```python
from build123d import *

# Parameters (mm, degrees)
SKETCH1_W                      = 200
SKETCH1_H                      = 300
BOSS_EXTRUDE1_DEPTH            = 4.7625
CUT_EXTRUDE1_DEPTH             = 181.340459704
SKETCH15_R                     = 3.5
BOSS_EXTRUDE2_DEPTH            = 4.7625
M3X0_5_TAPPED_HOLE3_D          = 2.5
M5_CLEARANCE_HOLE1_D           = 5.3
FILLET2_R                      = 3
M3X0_5_TAPPED_HOLE4_AT_2_COUNT = 2
M3X0_5_TAPPED_HOLE4_AT_2_PITCH = 150
M3X0_5_TAPPED_HOLE5_AT_2_COUNT = 2
M3X0_5_TAPPED_HOLE5_AT_2_PITCH = 137.5
M3X0_5_TAPPED_HOLE5_AT_3_COUNT = 2
M3X0_5_TAPPED_HOLE5_AT_3_PITCH = 275
FILLET1_R                      = 1


with BuildPart() as part:
    # Sketch1 → Boss-Extrude1 (new body)
    with BuildSketch(Plane(origin=(0, 0, 0), x_dir=(1, 0, 0), z_dir=(0, 1, 0))):
        Rectangle(SKETCH1_W, SKETCH1_H)
    extrude(amount=BOSS_EXTRUDE1_DEPTH)

    # Sketch14 → Cut-Extrude1 (cut, through all)
    with BuildSketch(Plane(origin=(0, 4.7625, 0), x_dir=(1, 0, 0), z_dir=(0, 1, 0))):
        Polygon((-83.751800259, 15), (83.751800259, 15), (0, -54.793166883), align=None)
        Polygon((90, 9.793166883), (90, -129.793166883), (6.248199741, -60), align=None)
        Polygon((83.751800259, -135), (-83.751800259, -135), (0, -65.206833117), align=None)
        Polygon((-90, -129.793166883), (-90, 9.793166883), (-6.248199741, -60), align=None)
        with BuildLine():
            Line((8.236504113, 90), (90, 135.424164382))
            Line((90, 135.424164382), (90, 128))
            ThreePointArc((90, 128), (87, 125), (90, 122))
            Line((90, 122), (90, 70))
            ThreePointArc((90, 70), (87, 67), (90, 64))
            Line((90, 64), (90, 44.575835618))
            Line((90, 44.575835618), (59.796175629, 61.355738047))
            Line((59.796175629, 61.355738047), (62.122471828, 65.543071206))
            ThreePointArc((62.122471828, 65.543071206), (60.956928794, 69.622471828), (56.877528172, 68.456928794))
            Line((56.877528172, 68.456928794), (54.551231972, 64.269595634))
            Line((54.551231972, 64.269595634), (8.236504113, 90))
        make_face()
        Polygon((81.763495887, 140), (0, 94.575835618), (-81.763495887, 140), align=None)
        Polygon((-90, 135.424164382), (-8.236504113, 90), (-90, 44.575835618), align=None)
        Polygon((-81.763495887, 40), (0, 85.424164382), (81.763495887, 40), align=None)
    extrude(amount=-CUT_EXTRUDE1_DEPTH, mode=Mode.SUBTRACT)

    # Sketch15 → Boss-Extrude2 (add)
    with BuildSketch(Plane(origin=(0, 4.7625, 0), x_dir=(1, 0, 0), z_dir=(0, 1, 0))):
        with Locations((85, -140)):
            Circle(SKETCH15_R)
    extrude(amount=-BOSS_EXTRUDE2_DEPTH)

    # M3x0.5 Tapped Hole3 (through all)
    with Locations(Plane(origin=(0, 4.7625, 0), x_dir=(1, 0, 0), z_dir=(0, 1, 0))):
        with Locations((85, 17.25), (-47, 17.25), (85, -140), (-70, -140), (-92, 145), (-92, 35), (43, 35), (43, 145), (59.5, 67), (90, 67), (90, 125), (59.5, 125)):
            Hole(M3X0_5_TAPPED_HOLE3_D / 2)

    # M5 Clearance Hole1 (through all)
    with Locations(Plane(origin=(0, 4.7625, 0), x_dir=(1, 0, 0), z_dir=(0, 1, 0))):
        with Locations((-95, 62.5), (-95, -62.5), (95, -62.5), (95, 62.5)):
            Hole(M5_CLEARANCE_HOLE1_D / 2)

    # Sketch29 → CSK for M5 Flat Head Machine Screw1 (revolve, cut)
    with BuildSketch(Plane(origin=(95, 4.7625, 62.5), x_dir=(0, 0, 1), z_dir=(1, 0, 0))):
        Polygon((0, 0), (0, 4.7625), (2.65, 4.7625), (2.65, 2.55), (5.2, 0), align=None)
    revolve(axis=Axis((95, 11.1125, 62.5), (0, -1, 0)), mode=Mode.SUBTRACT)

    # Fillet2
    fillet2_edges = [part.edges().sort_by_distance(p)[0] for p in [
        (6.248199741, 2.38125, 60),
        (90, 2.38125, -9.793166883),
        (90, 2.38125, 129.793166883),
        (54.551231972, 2.38125, -64.269595634),
        (8.236504113, 2.38125, -90),
        (90, 2.38125, -135.424164382),
        (90, 2.38125, -128),
        (90, 2.38125, -122),
        (90, 2.38125, -70),
        (90, 2.38125, -64),
        (90, 2.38125, -44.575835618),
        (59.796175629, 2.38125, -61.355738047),
        (-6.248199741, 2.38125, 60),
        (-90, 2.38125, 129.793166883),
        (-90, 2.38125, -9.793166883),
        (0, 2.38125, 54.793166883),
        (-83.751800259, 2.38125, -15),
        (83.751800259, 2.38125, -15),
        (0, 2.38125, 65.206833117),
        (83.751800259, 2.38125, 135),
        (-83.751800259, 2.38125, 135),
        (81.763495887, 2.38125, -40),
        (-81.763495887, 2.38125, -40),
        (0, 2.38125, -85.424164382),
        (-90, 2.38125, -44.575835618),
        (-90, 2.38125, -135.424164382),
        (-8.236504113, 2.38125, -90),
        (-81.763495887, 2.38125, -140),
        (81.763495887, 2.38125, -140),
        (0, 2.38125, -94.575835618),
    ]]
    fillet(fillet2_edges, radius=FILLET2_R)

    # Sketch22 → M3x0.5 Tapped Hole4 (revolve, cut)
    with BuildSketch(Plane(origin=(-75, 2.38125, 150), x_dir=(0, -1, 0), z_dir=(1, 0, 0))):
        Polygon((0, 0), (0, 10.751075774), (1.25, 10), (1.25, 0), align=None)
    m3x0_5_tapped_hole4 = revolve(axis=Axis((-75, 2.38125, 156.35), (0, 0, -1)), mode=Mode.SUBTRACT)

    # M3x0.5 Tapped Hole4 at 2: M3x0.5 Tapped Hole4 ×2
    with Locations(*[(i * M3X0_5_TAPPED_HOLE4_AT_2_PITCH, 0, 0) for i in range(1, M3X0_5_TAPPED_HOLE4_AT_2_COUNT)]):
        add(m3x0_5_tapped_hole4, mode=Mode.SUBTRACT)

    # Mirror1: M3x0.5 Tapped Hole4 across plane
    add(m3x0_5_tapped_hole4.mirror(Plane.XY), mode=Mode.SUBTRACT)

    # Mirror1 copy 1 sketch → Mirror1 copy 1 (revolve, cut)
    with BuildSketch(Plane(origin=(75, 2.38125, -150), x_dir=(0, -1, 0), z_dir=(1, 0, 0))):
        Polygon((0, 0), (0, -10.751075774), (1.25, -10), (1.25, 0), align=None)
    revolve(axis=Axis((75, 2.38125, -156.35), (0, 0, -1)), mode=Mode.SUBTRACT)

    # Sketch25 → M3x0.5 Tapped Hole5 (revolve, cut)
    with BuildSketch(Plane(origin=(-100, 2.38125, -137.5), x_dir=(0, 0, 1), z_dir=(0, 1, 0))):
        Polygon((0, 0), (0, 10.751075774), (1.25, 10), (1.25, 0), align=None)
    m3x0_5_tapped_hole5 = revolve(axis=Axis((-106.35, 2.38125, -137.5), (1, 0, 0)), mode=Mode.SUBTRACT)

    # M3x0.5 Tapped Hole5 at 2: M3x0.5 Tapped Hole5 ×2
    with Locations(*[(0, 0, i * M3X0_5_TAPPED_HOLE5_AT_2_PITCH) for i in range(1, M3X0_5_TAPPED_HOLE5_AT_2_COUNT)]):
        add(m3x0_5_tapped_hole5, mode=Mode.SUBTRACT)

    # M3x0.5 Tapped Hole5 at 3: M3x0.5 Tapped Hole5 ×2
    with Locations(*[(0, 0, i * M3X0_5_TAPPED_HOLE5_AT_3_PITCH) for i in range(1, M3X0_5_TAPPED_HOLE5_AT_3_COUNT)]):
        add(m3x0_5_tapped_hole5, mode=Mode.SUBTRACT)

    # Mirror2: M3x0.5 Tapped Hole5 across plane
    add(m3x0_5_tapped_hole5.mirror(Plane(origin=(0, 0, 0), x_dir=(0, 0, 1), z_dir=(1, 0, 0))), mode=Mode.SUBTRACT)

    # Mirror2 copy 1 sketch → Mirror2 copy 1 (revolve, cut)
    with BuildSketch(Plane(origin=(100, 2.38125, 0), x_dir=(0, 0, 1), z_dir=(0, 1, 0))):
        Polygon((0, 0), (0, -10.751075774), (1.25, -10), (1.25, 0), align=None)
    revolve(axis=Axis((106.35, 2.38125, 0), (1, 0, 0)), mode=Mode.SUBTRACT)

    # Mirror2 copy 2 sketch → Mirror2 copy 2 (revolve, cut)
    with BuildSketch(Plane(origin=(100, 2.38125, 137.5), x_dir=(0, 0, 1), z_dir=(0, 1, 0))):
        Polygon((0, 0), (0, -10.751075774), (1.25, -10), (1.25, 0), align=None)
    revolve(axis=Axis((106.35, 2.38125, 137.5), (1, 0, 0)), mode=Mode.SUBTRACT)

    # Fillet1
    fillet1_edges = [part.edges().sort_by_distance(p)[0] for p in [
        (100, 2.38125, 150),
        (-100, 2.38125, 150),
        (-100, 2.38125, -150),
        (100, 2.38125, -150),
    ]]
    fillet(fillet1_edges, radius=FILLET1_R)


solid = part.part
```
Input: part model. Units: mm. Frame: model coordinates. A direction names the side the tool comes from. Coordinates: 2 decimals unless noted, no trailing zeros. Loops run counter-clockwise (first coordinate to the right, second up) from the corner with the lowest first, then second, coordinate; pieces in that order, holes last. Notation, with made-up numbers: M 52,25.5 L 93,25.5 A23 cw 93,41.5 Z; hole C -23,45.5 d8. An arc over 180 degrees is marked long. Answer in a Markdown table with one row per item.
1. First-contact query: pin 1 (2 mm diameter, centred on x = 75, y = 2.38, fed in from -Z); pin 2 (3 mm diameter, centred on x = 43, z = -35, fed in from +Y); pin 3 (1.5 mm diameter, centred on x = 59.5, z = -67, fed in from +Y). Flat tips, straight axial feed; report the tip coordinate or a pass-through.
Response:
| item | result |
|---|---|
| pin 1 | stops at z = -139.85 |
| pin 2 | stops at y = 4.76 |
| pin 3 | passes through |
2. Draft query along Z for faces 1 (the flat face through (-8, 4.762, -23)), 2 (the flat face through (48.74, 2.41, -112.5)). Return one class per face: pulls with the +Z half, pulls with the -Z half, needs draft (parallel to the pull), parting line crosses it, or undercut.
Response:
| item | result |
|---|---|
| face 1 | needs draft |
| face 2 | undercut |
3. Reachability of faces 3 (the conical face through (97.49, 2.37, 63.8)), 4 (the flat face through (74.143, 2.415, -53.385)) from +Z, -Z, +X, -X, +Y, -Y: full face, straight path, thin tool, end or side. Return the list, or none.
Response:
| item | result |
|---|---|
| face 3 | +Y |
| face 4 | +Y, -Y |
4. Material intervals for line 1 (X direction, y = 1.35, z = -48); line 2 (Y direction, x = -75, z = 145); line 3 (X direction, y = 3.1, z = -51), sorted ascending.
Response:
| item | result |
|---|---|
| line 1 | x = -100 to -89.49, -83.84 to -67.36, 67.36 to 83.84, 89.49 to 100 |
| line 2 | y = 0 to 1.13, 3.63 to 4.76 |
| line 3 | x = -100 to -90, -78.44 to -61.96, 61.96 to 78.44, 90 to 100 |
5. Section B-B, the plane x = 28. Output: boundary loops of the cut face in (y, z), then the cut area to 3 significant figures.
Response:
| item | result |
|---|---|
| outline | M 0,-150 L 4.76,-150 L 4.76,-140 L 0,-140 Z; M 0,-110.13 L 4.76,-110.13 L 4.76,-100.98 L 0,-100.98 Z; M 0,-79.02 L 4.76,-79.02 L 4.76,-69.87 L 0,-69.87 Z; M 0,-40 L 4.76,-40 L 4.76,-15 L 0,-15 Z; M 0,31.46 L 4.76,31.46 L 4.76,41.87 L 0,41.87 Z; M 0,78.13 L 4.76,78.13 L 4.76,88.54 L 0,88.54 Z; M 0,135 L 4.76,135 L 4.76,150 L 0,150 Z |
| area | 424 mm2 |
6. Section A-A, the plane z = 101.5. Output: boundary loops of the cut face in (x, y), then the cut area to 3 significant figures.
Response:
| item | result |
|---|---|
| outline | M -100,0 L -90,0 L -90,4.76 L -100,4.76 Z; M -56.05,0 L -43.55,0 L -43.55,4.76 L -56.05,4.76 Z; M 43.55,0 L 56.05,0 L 56.05,4.76 L 43.55,4.76 Z; M 90,0 L 100,0 L 100,4.76 L 90,4.76 Z |
| area | 214 mm2 |
